Autodesk Inventor part; units mm, degrees
ref_plane "YZ Plane" through (0, 0, 0) normal (1, 0, 0) x (0, 1, 0)
ref_plane "XZ Plane" through (0, 0, 0) normal (0, 1, 0) x (-1, 0, 0)
ref_plane "XY Plane" through (0, 0, 0) normal (0, 0, 1) x (1, 0, 0)
sketch "スケッチ1" plane through (0, 0, 0) normal (0, 0, 1) x (1, 0, 0)
  line L0 (0, 0) -> (90, 0)
  line L1 (90, 0) -> (90, -42.5)
  line L2 (90, -42.5) -> (152, -42.5)
  line L3 (152, -42.5) -> (152, 47.5)
  line L4 (152, 47.5) -> (90, 47.5)
  line L5 (90, 47.5) -> (90, 5)
  line L6 (90, 5) -> (0, 5)
  line L7 (0, 5) -> (0, 0)
  line L8 (0, 2.5) -> (152, 2.5) construction
  dimension "d0" = 5
  dimension "d1" = 152
  dimension "d2" = 90
  dimension "d3" = 90
revolve "回転1" add sketch "スケッチ1" angle 360 about axis through (0, 5, 0) along (0, -1, 0)
sketch "スケッチ2" plane through (0, 5, 0) normal (0, 1, 0) x (1, 0, 0)
  circle A0 centre (0, 0) radius 37.5
  circle A1 centre (0, 45.5) radius 4
  line L0 (0, 0) -> (0, 45.5) construction
  circle A2 centre (-45.5, 0) radius 4
  circle A3 centre (0, -45.5) radius 4
  circle A4 centre (45.5, 0) radius 4
  line L1 (0, 0) -> (26.7878, 64.6716) construction
  circle A5 centre (26.7878, 64.6716) radius 15
  circle A6 centre (0, 0) radius 70 construction
  circle A7 centre (-26.7878, 64.6716) radius 15
  circle A8 centre (-64.6716, 26.7878) radius 15
  circle A9 centre (-64.6716, -26.7878) radius 15
  circle A10 centre (-26.7878, -64.6716) radius 15
  circle A11 centre (26.7878, -64.6716) radius 15
  circle A12 centre (64.6716, -26.7878) radius 15
  circle A13 centre (64.6716, 26.7878) radius 15
  dimension "d18" = 140
  dimension "d6" = 45.5
  dimension "d7" = 8
  dimension "d8" = 75
  dimension "d11" = 360
  dimension "d16" = 22.5
  dimension "d17" = 30
  dimension "d21" = 360
extrude "押し出し1" cut sketch "スケッチ2" against normal up to next
fillet "フィレット1" radius 20 4 edges at (-152, 47.5, 0) (-152, -42.5, 0) (-90, 47.5, 0) (-90, -42.5, 0)
properties part number "車輪"
Model file for the job. Use its own axes, mm. A direction names the side the tool comes from. Give positions to 0.01 mm unless a question says otherwise; leave off trailing zeros. Write each loop counter-clockwise with the first axis right and the second up, starting at its lowest first coordinate (ties: lowest second). Pieces come first, ordered by that corner, then holes. Notation, with made-up numbers: (-16, 14) - (37, 14) arc R35 cw to (37, 53) - close; hole circle Ø9 at (-21, 52.25). An arc over 180 degrees is marked (long way). One line per question, with ' | ' between items. Start each with the question number.
(1) Wall check: line 1 along Z through (x, y) = (32, 37.5); line 2 along Z through (x, y) = (-70, 15); line 3 along X through (y, z) = (-31, -16.5). Give the ranges that are in metal, low to high. Write a range as from..to.
(2) Slice it at A-A on z = 0. Give the number of separate pieces and of enclosed holes in the cut face, plus the area to 3 significant figures.
(3) 3-axis set-ups, long thin cutter, end or side, ignore diameter. For faces 4 (the face through (41.53, 16.093, -79.845)), 5 (the face through (-1, 0, -39)), 6 (the face through (53.616, 2.535, 16.65)): which of +Z, -Z, +X, -X, +Y, -Y reach the whole face in a straight line?
(4) Two-plate mould, pull along X, no slides. Class faces 1 (the face through (24.835, 2.535, -79.544)), 2 (the face through (70.14, 2.85, 134.85)), 3 (the face through (-30, 47.5, 108)): +X half, -X half, draft (parallel to the pull), parting line (faces both ways), or undercut.
(5) Pin check, flat tips, straight feed: P1, Ø4, axis at y = -28, z = -18, coming from the +X side; P2, Ø24, axis at x = -26.79, z = -64.67, coming from the +Y side; P3, Ø12, axis at x = 91, y = -26, coming from the -Z side; P4, Ø8, axis at x = -100.5, y = 34.5, coming from the -Z side. Stop position of each tip, or through.
(6) Slice it at C-C on y = -6.5. Write the cut outline in (x, z).
Results below:
1) line 1: -145.85..-86.98, 86.98..145.85 | line 2: -134.92..-56.57, 56.57..134.92 | line 3: -149.19..-90.4, 90.4..149.19
2) separate pieces: 4 | enclosed holes: 0 | area: 10,900 mm^2
3) face 4: +Y | face 5: -Y | face 6: +Y, -Y
4) face 1: undercut | face 2: parting line | face 3: draft
5) P1: x = 150.69 | P2: through | P3: z = -125.77 | P4: z = -116.2
6) outline: circle Ø304 at (0, 0); hole circle Ø180 at (0, 0)
